Here's how the part is built. I have some questions about the finished solid (model axes, mm). Round coordinates to 2 decimals unless told otherwise and drop trailing zeros. Write each loop counter-clockwise with the first axis right and the second up, starting at its lowest first coordinate (ties: lowest second). Pieces come first, ordered by that corner, then holes. Notation, with made-up numbers: (85, 75.25) -> (101, 75.25) arc R18 ccw to (101, 98.25) -> close; hole circle Ø4 at (-32.75, 26). An arc over 180 degrees is marked (long way). Put each result on its own line as item: value. Start each with the question number.
1. Suppose I cut it at B-B (x = -6). Please give me the cut outline in (y, z).
2. Suppose I cut it at C-C (z = 0.55). Count the separate pieces of the cut face and the enclosed holes in it, then the cut area to 3 significant figures.
3. For pin 1 (1.5 mm diameter, centred on x = 79, z = 2.5, fed in from +Y); pin 2 (1.5 mm diameter, centred on y = 4.5, z = 2, fed in from +X); pin 3 (3.5 mm diameter, centred on x = 0, y = -6, fed in from +Z); pin 4 (4 mm diameter, centred on x = 0, y = 0, fed in from -Z), each with a flat end and sliding along its axis, tell me the tip position at first contact or that it passes through.
4. Suppose I cut it at A-A (y = 0). Please give me the cut outline in (x, z).
5. I need wall thicknesses on probe 1 along Y at (x, z) = (0, 2.05); probe 2 along Y at (x, z) = (50, 0.65); probe 3 along X at (y, z) = (-6, 0.9). Which ranges of each line are inside material? Lowest first, please. Write a range as from..to.
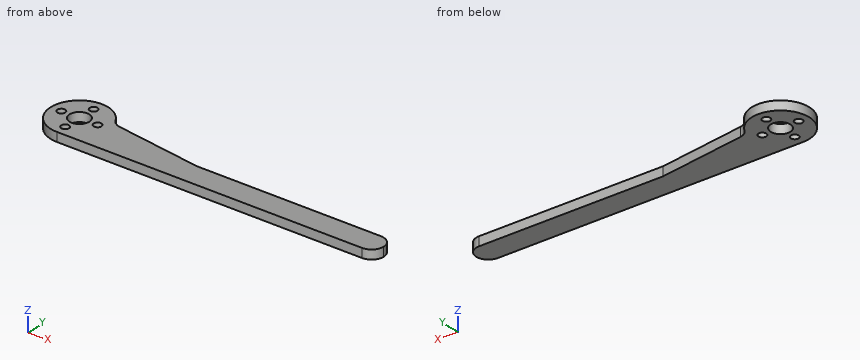
```python
from build123d import *

# Parameters (mm, degrees)
ESQUISSE1_R        = 9.5
ESQUISSE1_R_2      = 1.3
ESQUISSE1_R_3      = 3.25
BOSS_EXTRU_1_DEPTH = 3
BOSS_EXTRU_2_DEPTH = 3
ESQUISSE3_W        = 65
ESQUISSE3_H        = 8
BOSS_EXTRU_3_DEPTH = 3
CONG_1_R           = 4


with BuildPart() as part:
    # Esquisse1 → Boss.-Extru.1 (new body)
    with BuildSketch(Plane.XY):
        Circle(ESQUISSE1_R)
        with Locations((6, 0)):
            Circle(ESQUISSE1_R_2, mode=Mode.SUBTRACT)
        with Locations((0, 6)):
            Circle(ESQUISSE1_R_2, mode=Mode.SUBTRACT)
        with Locations(Location((-6, 0, 0), (0, 0, 180))):
            Circle(ESQUISSE1_R_2, mode=Mode.SUBTRACT)
        with Locations(Location((0, -6, 0), (0, 0, 180))):
            Circle(ESQUISSE1_R_2, mode=Mode.SUBTRACT)
        Circle(ESQUISSE1_R_3, mode=Mode.SUBTRACT)
    extrude(amount=BOSS_EXTRU_1_DEPTH)

    # Esquisse2 → Boss.-Extru.2 (add)
    with BuildSketch(Plane.XY.offset(3)):
        Polygon((0, -9.5), (40, -9.5), (40, -1.5), (9, 3.041381265), (9, -0.5), align=None)
    extrude(amount=-BOSS_EXTRU_2_DEPTH)

    # Esquisse3 → Boss.-Extru.3 (add)
    with BuildSketch(Plane.XY.offset(3)):
        with Locations((72.5, -5.5)):
            Rectangle(ESQUISSE3_W, ESQUISSE3_H)
    extrude(amount=-BOSS_EXTRU_3_DEPTH)

    # Congé1
    cong_1_edges = [part.edges().sort_by_distance(p)[0] for p in [
        (9, 3.041381265, 1.5),
        (105, -9.5, 1.5),
        (105, -1.5, 1.5),
    ]]
    fillet(cong_1_edges, radius=CONG_1_R - 0.0001)  # a hair under: the kernel refuses the full size


solid = part.part
```
Verdict:
1. outline: (-7.37, 0) -> (-1.3, 0) -> (-1.3, 3) -> (-7.37, 3) -> close; (1.3, 0) -> (7.37, 0) -> (7.37, 3) -> (1.3, 3) -> close
2. separate pieces: 1
2. enclosed holes: 5
2. area: 1,070 mm^2
3. pin 1: stops at y = -1.5
3. pin 2: stops at x = 9.01
3. pin 3: stops at z = 3
3. pin 4: passes through
4. outline: (-9.5, 0) -> (-7.3, 0) -> (-7.3, 3) -> (-9.5, 3) -> close; (-4.7, 0) -> (-3.25, 0) -> (-3.25, 3) -> (-4.7, 3) -> close; (3.25, 0) -> (4.7, 0) -> (4.7, 3) -> (3.25, 3) -> close; (7.3, 0) -> (29.76, 0) -> (29.76, 3) -> (7.3, 3) -> close
5. probe 1: y = -9.5..-7.3, -4.7..-3.25, 3.25..4.7, 7.3..9.5
5. probe 2: y = -9.5..-1.5
5. probe 3: x = -7.37..-1.3, 1.3..104.97
